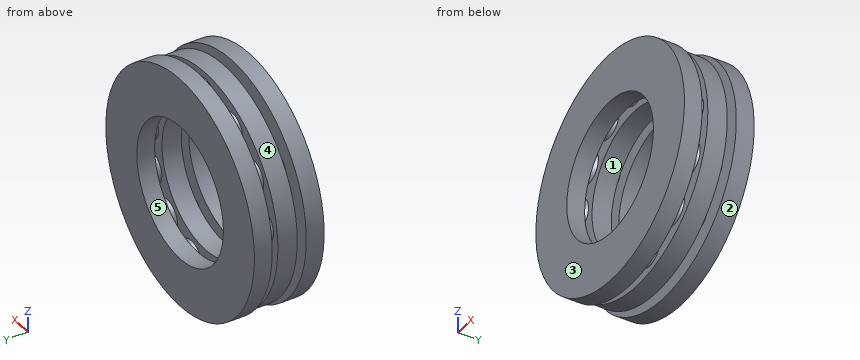
from build123d import *

# Parameters (mm, degrees)
F0_R     = 14.65
F0_R_2   = 8.75
F1_DEPTH = 1.25
F4_COUNT = 13
F5_W     = 2.3
F5_H     = 6.25


with BuildPart() as f1:
    # F0 (on Front) → F1 (new body, symmetric)
    with BuildSketch(Plane.XZ):
        Circle(F0_R)
        Circle(F0_R_2, mode=Mode.SUBTRACT)
    extrude(amount=F1_DEPTH, both=True)

    # F2 (on Front) → F3 (revolve)
    with BuildSketch(Plane.XZ):
        with BuildLine():
            Line((0, 14.2), (0, 9.2))
            ThreePointArc((0, 9.2), (2.5, 11.7), (0, 14.2))
        make_face()
    revolve(axis=Axis((0, 0, 11.7), (0, 0, -1)))

    # F4: F1 ×13 about axis
    f4_axis = Axis((0, -1.25, 0), (0, -1, 0))


with BuildPart() as f1_1:
    add(f1.part)
    for i in range(1, F4_COUNT):
        add(f1.part.rotate(f4_axis, i * 360 / F4_COUNT))

    # F5 (on Right) → F6 (revolve)
    with BuildSketch(Plane.YZ):
        with Locations((3.35, 11.875)):
            Rectangle(F5_W, F5_H)
        with Locations((-3.35, 11.875)):
            Rectangle(F5_W, F5_H)
    revolve(axis=Axis((0, 2.25, 0), (0, 1, 0)))


solid = f1_1.part
Check sheet for the modelled part. Datum: model origin and axes. Units: mm. Face numbers are marked on the shaded views. A direction names the side the tool comes from. Round coordinates to 2 decimals unless told otherwise and drop trailing zeros. Loops run counter-clockwise (first coordinate to the right, second up) from the corner with the lowest first, then second, coordinate; pieces in that order, holes last. Notation, with made-up numbers: M 58,16 L 116,16 A19 ccw 116,39 Z; hole C -37.75,42.25 d7. An arc over 180 degrees is marked long. One line per question, with ' | ' between items. Start each with the question number.
Item 1: Section check B-B (y = 3.25). Record the boundary of the cut face in (x, z), and give its area (3 significant figures).
Item 2: Release check for a two-part mould opening along X. For the marked faces 1, 2 and 3 record: released by +X, released by -X, zero draft, split by the parting line, or undercut.
Item 3: Set-up check for the marked faces 4 and 5: record each of +Z, -Z, +X, -X, +Y, -Y from which the full face is reachable in a straight line by a thin tool's end or side.
Item 4: Gauge pin test, flat ends, axial feed: pin 1 Ø1.5 at (y, z) = (0, -12) entering from -X; pin 2 Ø3 at (x, y) = (8, -2) entering from -Z; pin 3 Ø2 at (x, y) = (-4, -2) entering from -Z; pin 4 Ø14 at (x, z) = (0, 0) entering from -Y. Record the tip position at first contact, or that the pin passes through.
Item 5: Section check A-A (x = 0). State how many separate pieces and enclosed holes the cut face has, and give its area (3 significant figures).
Item 6: Scan lines: probe 1 along Z at (x, y) = (0, -0.7); probe 2 along Y at (x, z) = (-2, -9); probe 3 along Z at (x, y) = (6.5, -3.25). Record each from-to range of solid material in increasing order.
Item 7: Section check C-C (y = -0.5). Record the boundary of the cut face in (x, z).
Worked out:
1) outline: C 0,0 d30; hole C 0,0 d17.5 | area: 466 mm^2
2) face 1: undercut | face 2: split by the parting line | face 3: zero draft
3) face 4: none | face 5: +Y, -Y
4) pin 1: x = -9.38 | pin 2: z = -13.51 | pin 3: z = -14.69 | pin 4: through
5) separate pieces: 4 | enclosed holes: 0 | area: 93.7 mm^2
6) probe 1: -14.65 to -8.75, 8.75 to 14.65 | probe 2: -4.5 to -2.2, -1.25 to 1.25, 2.2 to 4.5 | probe 3: -13.52 to -5.86, 5.86 to 13.52
7) outline: C 0,0 d29.3; hole C 0,0 d17.5
